```python
from build123d import *

# Parameters (mm, degrees)
F0_R     = 7
F1_DEPTH = 10
F2_DEPTH = 10.001
F3_R     = 9.99999
F4_SIZE  = 1
F5_R     = 7
F6_DEPTH = 80


# Not quite as in the source:
# - a fillet or chamfer is up to 0.001 mm smaller than in the source, because OpenCascade refuses the exact size


with BuildPart() as f1:
    # F0 (on Top) → F1 (new body)
    with BuildSketch(Plane.XY):
        with BuildLine():
            Line((0, -20), (0, 0))
            Line((0, 0), (-137.6794919243, 0))
            ThreePointArc((-137.6794919243, 0), (-135.6814834742, -4.8236190979), (-135, -10))
            ThreePointArc((-135, -10), (-135.6814834742, -15.1763809021), (-137.6794919243, -20))
            Line((-137.6794919243, -20), (0, -20))
        make_face()
        with Locations((-10, -10)):
            Circle(F0_R, mode=Mode.SUBTRACT)
        with BuildLine():
            Line((-143.8196601125, 0), (-137.6794919243, 0))
            ThreePointArc((-137.6794919243, 0), (-175, -10), (-137.6794919243, -20))
            Line((-137.6794919243, -20), (-143.8196601125, -20))
            ThreePointArc((-143.8196601125, -20), (-170, -10), (-143.8196601125, 0))
        make_face()
        with BuildLine():
            ThreePointArc((-135, -10), (-135.6814834742, -4.8236190979), (-137.6794919243, 0))
            Line((-137.6794919243, 0), (-143.8196601125, 0))
            ThreePointArc((-143.8196601125, 0), (-140.9874146156, -4.6476686534), (-140, -10))
            ThreePointArc((-140, -10), (-140.9874146156, -15.3523313466), (-143.8196601125, -20))
            Line((-143.8196601125, -20), (-137.6794919243, -20))
            ThreePointArc((-137.6794919243, -20), (-135.6814834742, -15.1763809021), (-135, -10))
        make_face()
    extrude(amount=F1_DEPTH)

    # F0 (on Top) → F2 (cut, through all)
    with BuildSketch(Plane.XY):
        with BuildLine():
            Line((-165, 0), (-143.8196601125, 0))
            ThreePointArc((-143.8196601125, 0), (-170, -10), (-143.8196601125, -20))
            Line((-143.8196601125, -20), (-165, -20))
            Line((-165, -20), (-165, 0))
        make_face()
        with BuildLine():
            ThreePointArc((-140, -10), (-140.9874146156, -4.6476686534), (-143.8196601125, 0))
            Line((-143.8196601125, 0), (-165, 0))
            Line((-165, 0), (-165, -20))
            Line((-165, -20), (-143.8196601125, -20))
            ThreePointArc((-143.8196601125, -20), (-140.9874146156, -15.3523313466), (-140, -10))
        make_face()
        with Locations((-10, -10)):
            Circle(F0_R)
    extrude(amount=F2_DEPTH, mode=Mode.SUBTRACT)

    # F3 (radius 10 in the source; OpenCascade refuses exactly that, so slightly less here)
    f3_edges = [f1.edges().sort_by_distance(p)[0] for p in [
        (0, -20, 5),
        (0, 0, 5),
        (-137.679492, -20, 5),
        (-137.679492, 0, 5),
    ]]
    fillet(f3_edges, radius=F3_R)

    # F4
    f4_edges = [f1.edges().sort_by_distance(p)[0] for p in [
        (-71.319657, -20, 0),
        (-2.928929, -2.928929, 10),
        (-71.319657, -20, 10),
        (-136.721804, -20.87129, 0),
        (-2.928929, -17.071071, 0),
        (-175, -10, 0),
        (0, -10, 0),
        (-136.721804, 0.87129, 0),
        (-2.928929, -2.928929, 0),
        (-71.319657, 0, 0),
        (-136.721804, -20.87129, 10),
        (-2.928929, -17.071071, 10),
        (-175, -10, 10),
        (0, -10, 10),
        (-136.721804, 0.87129, 10),
        (-71.319657, 0, 10),
    ]]
    chamfer(f4_edges, length=F4_SIZE)

    # F5 (on face) → F6 (join)
    with BuildSketch(Plane.XY.offset(10)):
        with Locations((-10, -10)):
            Circle(F5_R)
    extrude(amount=-F6_DEPTH)


solid = f1.part
```
The listing builds one solid part. Answer for the finished solid, in the listing's coordinates (mm). A direction names the side the tool comes from. Coordinates: 2 decimals unless noted, no trailing zeros. Loops run counter-clockwise (first coordinate to the right, second up) from the corner with the lowest first, then second, coordinate; pieces in that order, holes last. Notation, with made-up numbers: M 40,-3 L 49,-3 A16 cw 49,1 Z; hole C 54.25,6.5 d3. An arc over 180 degrees is marked long. Answer as a JSON object with one key per item and string values. Group by question number.
Item 1: Determine the mould class of faces 1 (the face through (-137, 1, 5)), 2 (the face through (-2.85, -16.99, 5.06)), 3 (the face through (-10, -10, -70)), 4 (the face through (-3.534, -12.681, -34.51)) for opening direction Y: +Y half, -Y half, draft (parallel to the pull), parting line (faces both ways), or undercut.
Item 2: Which of the six approach directions +Z, -Z, +X, -X, +Y, -Y give full straight-line access (tool end or side, diameter ignored) to faces 5 (the face through (-72, -20, 5)), 6 (the face through (-89, -10, 10)), 7 (the face through (-70, 0, 5))?
Item 3: Section A-A (x = -155) is taken. Write down the section's boundary in (y, z).
Item 4: Each of these flat-tipped pins is pushed along its axis until it touches: P1, Ø2.5, axis at x = -75, z = 5.5, coming from the -Y side; P2, Ø4, axis at x = -64.5, z = 3, coming from the +Y side; P3, Ø8, axis at y = -3.5, z = -42, coming from the +X side. Where does it stop, or does it pass through?
Item 5: Section C-C (x = -101) is taken. Write down the section's boundary in (y, z), and give its area (3 significant figures).
Item 6: Section D-D (z = -59.5) is taken. Write down the section's boundary in (x, y), and give its area (3 significant figures).
Item 7: Consider L1, parallel to Y at x = -155, z = 2.5; L2, parallel to Z at x = -116, y = -6.5; L3, parallel to Y at x = -152, z = 3.5. Determine where each line is inside the solid, lowest interval first.
Solved:
{
 "1": {"face 1": "+Y half", "face 2": "-Y half", "face 3": "draft", "face 4": "parting line"},
 "2": {"face 5": "+Z, -Z, +X, -Y", "face 6": "+Z, +X, -X, +Y, -Y", "face 7": "+Z, -Z, +X, +Y"},
 "3": {"outline": "M -30,1 L -29,0 L -25,0 L -25,10 L -29,10 L -30,9 Z; M 5,0 L 9,0 L 10,1 L 10,9 L 9,10 L 5,10 Z"},
 "4": {"P1": "stops at y = -20", "P2": "stops at y = 0", "P3": "stops at x = -3.46"},
 "5": {"outline": "M -20,1 L -19,0 L -1,0 L 0,1 L 0,9 L -1,10 L -19,10 L -20,9 Z", "area": "198 mm2"},
 "6": {"outline": "C -10,-10 d14", "area": "154 mm2"},
 "7": {"L1": "y = -30 to -25, 5 to 10", "L2": "z = 0 to 10", "L3": "y = -29.77 to -24.7, 4.7 to 9.77"}
}
